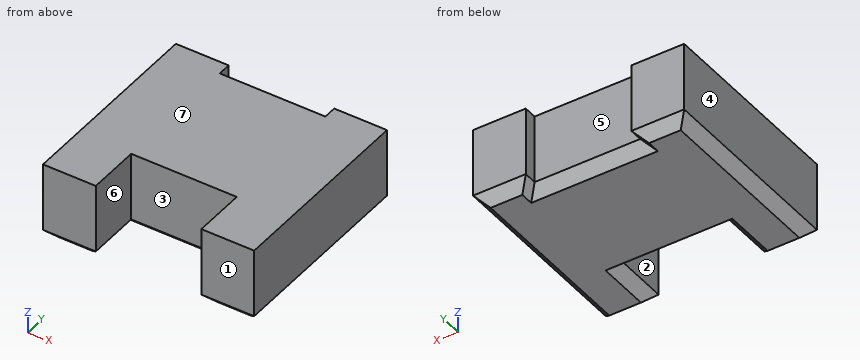
from build123d import *

# Parameters (mm, degrees)
PAD_DEPTH    = 3
CHAMFER_SIZE = 0.4


with BuildPart() as part:
    # Sketch → Pad (new body)
    with BuildSketch(Plane.XY):
        Polygon((-2, -2), (-2, 0), (2, 0), (2, -2), (4, -2), (4, 5.5), (2, 5.5), (2, 5), (-2, 5), (-2, 5.5), (-4, 5.5), (-4, -2), align=None)
    extrude(amount=PAD_DEPTH)

    # Chamfer
    chamfer_edges = [part.edges().sort_by_distance(p)[0] for p in [
        (-4, 1.75, 0),
        (-3, -2, 0),
        (-2, -1, 0),
        (0, 0, 0),
        (2, -1, 0),
        (3, -2, 0),
        (4, 1.75, 0),
        (3, 5.5, 0),
        (2, 5.25, 0),
        (0, 5, 0),
        (-2, 5.25, 0),
        (-3, 5.5, 0),
    ]]
    chamfer(chamfer_edges, length=CHAMFER_SIZE)


solid = part.part
Part model, mm, in its own coordinate system. Face numbers are marked on the shaded views. A direction names the side the tool comes from. Give positions to 0.01 mm unless a question says otherwise; leave off trailing zeros. Order: outer loops, then holes, each group sorted by start corner. A loop starts at its lowest first (then second) coordinate and runs counter-clockwise, first axis right, second up. Notation, with made-up numbers: (-17.75, 37) - (-13.75, 37) arc R8 ccw to (-13.75, 51) - close; hole circle Ø2 at (72.25, 81). An arc over 180 degrees is marked (long way). One line per question, with ' | ' between items.
1. Drop a flat-ended pin along its axis: P1, Ø1.3, axis at x = -0.5, z = 2, coming from the -Y side. Give the stop position or say it passes through.
Filled in:
P1: y = 0
2. Band-saw the part on A-A on z = 2.2. List the corners of the cut face in (x, y).
Filled in:
outline: (-4, -2) - (-2, -2) - (-2, 0) - (2, 0) - (2, -2) - (4, -2) - (4, 5.5) - (2, 5.5) - (2, 5) - (-2, 5) - (-2, 5.5) - (-4, 5.5) - close
3. Drill centre lines: probe 1 along X at (y, z) = (-1.5, 2.25); probe 2 along Y at (x, z) = (1, 2.5); probe 3 along Z at (x, y) = (-3, 5.25). Where is each one in solid material? Low to high.
Filled in:
probe 1: -4 to -2, 2 to 4 | probe 2: 0 to 5 | probe 3: 0.15 to 3
4. Band-saw the part on B-B on x = 1.5. List the corners of the cut face in (y, z), then the cut area to 3 significant figures.
Filled in:
outline: (0, 0.4) - (0.4, 0) - (4.6, 0) - (5, 0.4) - (5, 3) - (0, 3) - close | area: 14.8 mm²
5. Which spindle directions (+Z, -Z, +X, -X, +Y, -Y) get a long thin tool onto all of the face, cutting with end or side? Do the marked faces 5, 6 and 7. Say none if no direction does.
Filled in:
face 5: +Z, -Z, +Y | face 6: +Z, -Z, -Y | face 7: +Z, +X, -X, +Y, -Y
6. Pull direction X, two halves, no side cores. Call the marked faces 1, 2, 3 and 4: +X half, -X half, draft (parallel to the pull), parting line (faces both ways), or undercut.
Filled in:
face 1: draft | face 2: undercut | face 3: undercut | face 4: -X half
